from build123d import *

# Parameters (mm, degrees)
SKETCH1_W                 = 58
SKETCH1_H                 = 24
BOSS_EXTRUDE1_DEPTH       = 30
F_8_32_TAPPED_HOLE2_D     = 3.4544
F_8_32_TAPPED_HOLE2_DEPTH = 12
F_8_32_TAPPED_HOLE2_TIP   = 1.037806461
SKETCH18_W                = 41.2
SKETCH18_H                = 20.2
CUT_EXTRUDE6_DEPTH        = 28
SKETCH22_R                = 1.505
CUT_EXTRUDE9_DEPTH        = 2
SKETCH24_W                = 10.02
SKETCH24_H                = 10.02
CUT_EXTRUDE11_DEPTH       = 2
FILLET1_R                 = 10
FILLET2_R                 = 10
FILLET3_R                 = 10
FILLET4_R                 = 10


with BuildPart() as part:
    # Sketch1 → Boss-Extrude1 (new body)
    with BuildSketch(Plane.XY):
        Rectangle(SKETCH1_W, SKETCH1_H)
    extrude(amount=-BOSS_EXTRUDE1_DEPTH)

    # #8-32 Tapped Hole2
    with Locations(Plane(origin=(24.4, -5, 0), x_dir=(1, 0, 0), z_dir=(0, 0, 1))):
        with Locations((0, 0), (0, 10), (-48.8, 0), (-48.8, 10)):
            Hole(F_8_32_TAPPED_HOLE2_D / 2, depth=F_8_32_TAPPED_HOLE2_DEPTH)
            with Locations((0, 0, -(F_8_32_TAPPED_HOLE2_DEPTH + F_8_32_TAPPED_HOLE2_TIP / 2))):  # 118° drill point
                Cone(0, F_8_32_TAPPED_HOLE2_D / 2, F_8_32_TAPPED_HOLE2_TIP, mode=Mode.SUBTRACT)

    # Sketch18 → Cut-Extrude6 (cut)
    with BuildSketch(Plane.XY):
        Rectangle(SKETCH18_W, SKETCH18_H)
    extrude(amount=-CUT_EXTRUDE6_DEPTH, mode=Mode.SUBTRACT)

    # Sketch22 → Cut-Extrude9 (cut)
    with BuildSketch(Plane(origin=(0, 0, -30), x_dir=(-1, 0, 0), z_dir=(0, 0, -1))):
        with Locations((10.5, 0)):
            Circle(SKETCH22_R)
    extrude(amount=-CUT_EXTRUDE9_DEPTH, mode=Mode.SUBTRACT)

    # Sketch24 → Cut-Extrude11 (cut)
    with BuildSketch(Plane(origin=(0, -10.1, 0), x_dir=(1, 0, 0), z_dir=(0, 1, 0))):
        with Locations((-10.5, 6.6)):
            Rectangle(SKETCH24_W, SKETCH24_H)
    extrude(amount=-CUT_EXTRUDE11_DEPTH, mode=Mode.SUBTRACT)

    # Fillet1
    fillet1_edges = [part.edges().sort_by_distance(p)[0] for p in [
        (-29, 12, -15),
    ]]
    fillet(fillet1_edges, radius=FILLET1_R)

    # Fillet2
    fillet2_edges = [part.edges().sort_by_distance(p)[0] for p in [
        (29, 12, -15),
    ]]
    fillet(fillet2_edges, radius=FILLET2_R)

    # Fillet3
    fillet3_edges = [part.edges().sort_by_distance(p)[0] for p in [
        (29, -12, -15),
    ]]
    fillet(fillet3_edges, radius=FILLET3_R)

    # Fillet4
    fillet4_edges = [part.edges().sort_by_distance(p)[0] for p in [
        (-29, -12, -15),
    ]]
    fillet(fillet4_edges, radius=FILLET4_R)


solid = part.part
Could you check a few things on this model? Use its own coordinates, in mm. A direction names the side the tool comes from. Give positions to 0.01 mm unless a question says otherwise; leave off trailing zeros. Order: outer loops, then holes, each group sorted by start corner. A loop starts at its lowest first (then second) coordinate and runs counter-clockwise, first axis right, second up. Notation, with made-up numbers: M 0.5,-19 L 38.5,-19 A27 ccw 38.5,17 Z; hole C -17.5,2 d1. An arc over 180 degrees is marked long. One line per question, with ' | ' between items.
1. We'd pull the mould along Z, two halves only. Please class faces 1 (the face through (20.6, 0, -14)), 2 (the face through (-11, -11, -1.59)), 3 (the face through (24.162, -5.183, -12.858)): +Z half, -Z half, draft (parallel to the pull), parting line (faces both ways), or undercut.
Results:
face 1: draft | face 2: undercut | face 3: +Z half
2. I want a section at D-D (x = 18). List the corners of the cut face in (y, z) for me, and give its area (3 significant figures).
Results:
outline: M -12,-30 L 12,-30 L 12,0 L 10.1,0 L 10.1,-28 L -10.1,-28 L -10.1,0 L -12,0 Z | area: 154 mm²
3. I want a section at A-A (y = 0). List the corners of the cut face in (x, z) for me (3 decimals), and give its area (3 significant figures).
Results:
outline: M -29,-30 L -12.005,-30 L -12.005,-28 L -20.6,-28 L -20.6,0 L -29,0 Z; M -8.995,-30 L 29,-30 L 29,0 L 20.6,0 L 20.6,-28 L -8.995,-28 Z | area: 580 mm²
4. I'm going to push flat-ended pins straight in: pin 1 (1.5 mm diameter, centred on y = -10.5, z = -5, fed in from +X); pin 2 (8 mm diameter, centred on y = -6.5, z = -13.5, fed in from -X); pin 3 (3 mm diameter, centred on x = -24.4, y = 5, fed in from +Z). Where does each tip first touch, or does it pass through?
Results:
pin 1: x = 25.32 | pin 2: x = -28.99 | pin 3: z = -12.14
5. I want a section at B-B (z = -10.25). List the corners of the cut face in (x, y) for me.
Results:
outline: M -29,-2 A10 ccw -19,-12 L -15.51,-12 L -15.51,-10.1 L -20.6,-10.1 L -20.6,10.1 L 20.6,10.1 L 20.6,-10.1 L -5.49,-10.1 L -5.49,-12 L 19,-12 A10 ccw 29,-2 L 29,2 A10 ccw 19,12 L -19,12 A10 ccw -29,2 Z; hole C -24.4,-5 d3.45; hole C -24.4,5 d3.45; hole C 24.4,-5 d3.45; hole C 24.4,5 d3.45
6. If I drill on line 1 (Y direction, x = 13.5, z = -21.25); line 2 (Y direction, x = -24.4, z = -5); line 3 (X direction, y = 5.5, z = -1.75), over which ranges is the centre line in solid material (lowest first)?
Results:
line 1: -12 to -10.1, 10.1 to 12 | line 2: -10.42 to -6.73, -3.27 to 3.27, 6.73 to 10.42 | line 3: -28.37 to -26.05, -22.75 to -20.6, 20.6 to 22.75, 26.05 to 28.37
7. For faces 4 (the face through (-15.51, -11, -7)), 5 (the face through (-20.6, 0, -14)), 6 (the face through (-29, 0, -15)), which set-ups out of +Z, -Z, +X, -X, +Y, -Y let a thin tool reach every point of the face, with its end or its side?
Results:
face 4: -Y | face 5: +Z | face 6: +Z, -Z, -X, +Y, -Y
8. I want a section at C-C (z = -26.75). List the corners of the cut face in (x, y) for me, and give its area (3 significant figures).
Results:
outline: M -29,-2 A10 ccw -19,-12 L 19,-12 A10 ccw 29,-2 L 29,2 A10 ccw 19,12 L -19,12 A10 ccw -29,2 Z; hole M -20.6,-10.1 L 20.6,-10.1 L 20.6,10.1 L -20.6,10.1 Z | area: 474 mm²
